```python
from build123d import *

# Parameters (mm, degrees)
F0_R           = 6.4699981168
F1_DEPTH       = 10
F1_DEPTH_BACK  = 50
F1_FACE_R      = 6.4699981168
F2_DEPTH       = 5
F2_TAPER       = 10
F1_FACE1_R     = 6.4699981168
F3_DEPTH       = 5
F3_TAPER       = 10
F4_R           = 2.6340165395
F5_DEPTH       = 5
F5_TAPER       = -20
F6_R           = 3.8875838451
F7_DEPTH       = 5
F7_TAPER       = 20
F8_W           = 10.0221466273
F8_H           = 2.0072241314
F8_H_2         = 1.9136306364
F8_W_2         = 10.0826621056
F9_DEPTH       = 25
F10_R          = 6.2562819227
F11_DEPTH      = 10
F11_DEPTH_BACK = 50
F11_FACE_R     = 6.2562819227
F12_DEPTH      = 5
F12_TAPER      = 10
F11_FACE1_R    = 6.2562819227
F13_DEPTH      = 5
F13_TAPER      = 10
F14_R          = 2.2911639189
F15_DEPTH      = 5
F15_TAPER      = -20
F16_R          = 3.8569980959
F17_DEPTH      = 5
F17_TAPER      = 20
F18_R          = 6.6968336437
F19_DEPTH      = 10
F19_DEPTH_BACK = 50
F19_FACE_R     = 6.6968336437
F20_DEPTH      = 5
F20_TAPER      = 10
F19_FACE1_R    = 6.6968336437
F21_DEPTH      = 5
F21_TAPER      = 10
F22_R          = 2.6922121505
F23_DEPTH      = 5
F23_TAPER      = -20
F24_R          = 3.9459371666
F25_DEPTH      = 5
F25_TAPER      = 20
F26_DEPTH      = 30
F26_FACE_R     = 5.5883632132
F27_DEPTH      = 5
F27_TAPER      = -10
F28_DEPTH      = 10
F28_FACE_R     = 6.4699981168
F29_DEPTH      = 5
F29_TAPER      = 10
F29_FACE_R     = 5.5883632132
F30_DEPTH      = 3
F30_TAPER      = 15
F30_FACE_R     = 4.7845156359
F31_DEPTH      = 2
F31_TAPER      = 40
F31_FACE_R     = 3.1063163736
F32_DEPTH      = 1
F32_TAPER      = 50
F33_DEPTH      = 10
F33_FACE_R     = 1.914562781
F34_DEPTH      = 3
F34_TAPER      = 30


with BuildPart() as f1:
    # F0 (on Top) → F1 (new body, two sides)
    with BuildSketch(Plane.XY) as f1_sk:
        Circle(F0_R)
    extrude(amount=F1_DEPTH)
    extrude(f1_sk.sketch, amount=-F1_DEPTH_BACK)

    # F1_face (on face) → F2 (join)
    with BuildSketch(Plane.XY.offset(10)):
        Circle(F1_FACE_R)
    extrude(amount=F2_DEPTH, taper=F2_TAPER)

    # F1_face1 (on face) → F3 (join)
    with BuildSketch(Plane(origin=(0, 0, -50), x_dir=(1, 0, 0), z_dir=(0, 0, -1))):
        Circle(F1_FACE1_R)
    extrude(amount=F3_DEPTH, taper=F3_TAPER)

    # F4 (on face) → F5 (join)
    with BuildSketch(Plane(origin=(0, 0, -55), x_dir=(1, 0, 0), z_dir=(0, 0, -1))):
        Circle(F4_R)
    extrude(amount=F5_DEPTH, taper=F5_TAPER)

    # F6 (on face) → F7 (cut)
    with BuildSketch(Plane(origin=(0, 0, -60), x_dir=(1, 0, 0), z_dir=(0, 0, -1))):
        Circle(F6_R)
    extrude(amount=-F7_DEPTH, taper=F7_TAPER, mode=Mode.SUBTRACT)

    # F8 (on Top) → F9 (join)
    with BuildSketch(Plane.XY):
        with Locations((-5.0110733137, -1.0036120657)):
            Rectangle(F8_W, F8_H)
        with Locations((-5.0110733137, 0.9568153182)):
            Rectangle(F8_W, F8_H_2)
        with Locations((5.0413310528, 0.9568153182)):
            Rectangle(F8_W_2, F8_H_2)
        with Locations((5.0413310528, -1.0036120657)):
            Rectangle(F8_W_2, F8_H)
    extrude(amount=-F9_DEPTH)

    # F10 (on face) → F11 (join, two sides)
    with BuildSketch(Plane.XY) as f11_sk:
        with BuildLine():
            ThreePointArc((9.3005501419, -2.0072241314), (16.2432425413, -6.1730446317), (21.4823797001, 0))
            ThreePointArc((21.4823797001, 0), (16.1945878695, 6.1808648616), (9.269665852, 1.9136306364))
            Line((9.269665852, 1.9136306364), (10.0826621056, 1.9136306364))
            Line((10.0826621056, 1.9136306364), (10.0826621056, -2.0072241314))
            Line((10.0826621056, -2.0072241314), (9.3005501419, -2.0072241314))
        make_face()
        with Locations((15.2260977775, 0)):
            Circle(F10_R)
    extrude(amount=F11_DEPTH)
    extrude(f11_sk.sketch, amount=-F11_DEPTH_BACK)

    # F11_face (on face) → F12 (join)
    with BuildSketch(Plane(origin=(15.2260977775, 0, 10), x_dir=(1, 0, 0), z_dir=(0, 0, 1))):
        Circle(F11_FACE_R)
    extrude(amount=F12_DEPTH, taper=F12_TAPER)

    # F11_face1 (on face) → F13 (join)
    with BuildSketch(Plane(origin=(15.2260977775, 0, -50), x_dir=(1, 0, 0), z_dir=(0, 0, -1))):
        Circle(F11_FACE1_R)
    extrude(amount=F13_DEPTH, taper=F13_TAPER)

    # F14 (on face) → F15 (join)
    with BuildSketch(Plane(origin=(0, 0, -55), x_dir=(1, 0, 0), z_dir=(0, 0, -1))):
        with Locations((15.2260977775, 0)):
            Circle(F14_R)
    extrude(amount=F15_DEPTH, taper=F15_TAPER)

    # F16 (on face) → F17 (cut)
    with BuildSketch(Plane(origin=(0, 0, -60), x_dir=(1, 0, 0), z_dir=(0, 0, -1))):
        with Locations((15.2260977775, 0)):
            Circle(F16_R)
    extrude(amount=-F17_DEPTH, taper=F17_TAPER, mode=Mode.SUBTRACT)

    # F18 (on face) → F19 (join, two sides)
    with BuildSketch(Plane.XY) as f19_sk:
        with BuildLine():
            ThreePointArc((-8.7388105431, -2.0072241314), (-8.5083423849, -1.0153501193), (-8.4309229892, 0))
            ThreePointArc((-8.4309229892, 0), (-8.5010989129, 0.9669479373), (-8.7101559411, 1.9136306364))
            Line((-8.7101559411, 1.9136306364), (-10.0221466273, 1.9136306364))
            Line((-10.0221466273, 1.9136306364), (-10.0221466273, -2.0072241314))
            Line((-10.0221466273, -2.0072241314), (-8.7388105431, -2.0072241314))
        make_face()
        with Locations((-15.1277566329, 0)):
            Circle(F18_R)
    extrude(amount=F19_DEPTH)
    extrude(f19_sk.sketch, amount=-F19_DEPTH_BACK)

    # F19_face (on face) → F20 (join)
    with BuildSketch(Plane(origin=(-15.1277566329, 0, 10), x_dir=(1, 0, 0), z_dir=(0, 0, 1))):
        Circle(F19_FACE_R)
    extrude(amount=F20_DEPTH, taper=F20_TAPER)

    # F19_face1 (on face) → F21 (join)
    with BuildSketch(Plane(origin=(-15.1277566329, 0, -50), x_dir=(1, 0, 0), z_dir=(0, 0, -1))):
        Circle(F19_FACE1_R)
    extrude(amount=F21_DEPTH, taper=F21_TAPER)

    # F22 (on face) → F23 (join)
    with BuildSketch(Plane(origin=(0, 0, -55), x_dir=(1, 0, 0), z_dir=(0, 0, -1))):
        with Locations((-15.1277566329, 0)):
            Circle(F22_R)
    extrude(amount=F23_DEPTH, taper=F23_TAPER)

    # F24 (on face) → F25 (cut)
    with BuildSketch(Plane(origin=(0, 0, -60), x_dir=(1, 0, 0), z_dir=(0, 0, -1))):
        with Locations((-15.1277566329, 0)):
            Circle(F24_R)
    extrude(amount=-F25_DEPTH, taper=F25_TAPER, mode=Mode.SUBTRACT)

    # F26 (add): a face of the model
    f26_faces = [f1.faces().sort_by_distance(p)[0] for p in [
        (0, 0, 15),
    ]]
    extrude(f26_faces, amount=F26_DEPTH)

    # F26_face (on face) → F27 (join)
    with BuildSketch(Plane.XY.offset(45)):
        Circle(F26_FACE_R)
    extrude(amount=F27_DEPTH, taper=F27_TAPER)

    # F28 (add): a face of the model
    f28_faces = [f1.faces().sort_by_distance(p)[0] for p in [
        (0, 0, 50),
    ]]
    extrude(f28_faces, amount=F28_DEPTH)

    # F28_face (on face) → F29 (join)
    with BuildSketch(Plane.XY.offset(60)):
        Circle(F28_FACE_R)
    extrude(amount=F29_DEPTH, taper=F29_TAPER)

    # F29_face (on face) → F30 (join)
    with BuildSketch(Plane.XY.offset(65)):
        Circle(F29_FACE_R)
    extrude(amount=F30_DEPTH, taper=F30_TAPER)

    # F30_face (on face) → F31 (join)
    with BuildSketch(Plane.XY.offset(68)):
        Circle(F30_FACE_R)
    extrude(amount=F31_DEPTH, taper=F31_TAPER)

    # F31_face (on face) → F32 (join)
    with BuildSketch(Plane.XY.offset(70)):
        Circle(F31_FACE_R)
    extrude(amount=F32_DEPTH, taper=F32_TAPER)

    # F33 (add): a face of the model
    f33_faces = [f1.faces().sort_by_distance(p)[0] for p in [
        (0, 0, 71),
    ]]
    extrude(f33_faces, amount=F33_DEPTH)

    # F33_face (on face) → F34 (join)
    with BuildSketch(Plane.XY.offset(81)):
        Circle(F33_FACE_R)
    extrude(amount=F34_DEPTH, taper=F34_TAPER)


solid = f1.part
```
Geometry check sheet. Reference: the model listing, model coordinates, mm. A direction names the side the tool comes from. Round coordinates to 2 decimals unless told otherwise and drop trailing zeros. Order: outer loops, then holes, each group sorted by start corner. A loop starts at its lowest first (then second) coordinate and runs counter-clockwise, first axis right, second up. Notation, with made-up numbers: (-14.5, -4) - (30.5, -4) arc R17 cw to (30.5, 15) - close; hole circle Ø7 at (22, -3). An arc over 180 degrees is marked (long way). Use a Markdown table: item, result. Add a question column.
1) Section check B-B (z = 25). Record the cut outline in (x, y).
2) Set-up check for faces 4 (the flat face through (15, 0, 15)), 5 (the cylindrical face through (-0.25, -1.9, 75.93)), 6 (the flat face through (18, 0, -55)): record each of +Z, -Z, +X, -X, +Y, -Y from which the full face is reachable in a straight line by a thin tool's end or side.
3) Mould release check, pull along Z, two halves, no side actions. Record for faces 1 (the flat face through (-7, -2.007, -12)), 2 (the conical face through (-0.555, 2.5, -56.354)), 3 (the flat face through (-14, 3, -55)): released by +Z, released by -Z, zero draft, split by the parting line, or undercut.
4) Section check A-A (z = -16). Record the cut outline in (x, y).
5) Gauge pin test, flat ends, axial feed: P1, Ø4, axis at y = -4.5, z = -1.5, coming from the +X side; P2, Ø1.6, axis at x = 8, y = -0.5, coming from the +Z side; P3, Ø1.5, axis at x = -12, y = 4.5, coming from the +Z side; P4, Ø8, axis at x = 9.5, y = 3, coming from the -Z side. Record the tip position at first contact, or that the pin passes through.
6) Thickness scan on line 1 along X through (y, z) = (-0.5, -44); line 2 along X through (y, z) = (-3, -47.5); line 3 along Z through (x, y) = (-12, 2.5). Record the ranges inside material, lowest first.
Established:
| question | item | result |
|---|---|---|
| 1 | outline | circle Ø11.18 at (0, 0) |
| 2 | face 4 | +Z, +X, +Y, -Y |
| 2 | face 5 | +Z |
| 2 | face 6 | none |
| 3 | face 1 | zero draft |
| 3 | face 2 | released by -Z |
| 3 | face 3 | undercut |
| 4 | outline | (-8.74, -2.01) - (-6.15, -2.01) arc R6.47 ccw to (6.15, -2.01) - (9.3, -2.01) arc R6.26 ccw (long way) to (9.27, 1.91) - (6.18, 1.91) arc R6.47 ccw to (-6.18, 1.91) - (-8.71, 1.91) arc R6.7 ccw (long way) to start |
| 5 | P1 | x = 20.96 |
| 5 | P2 | z = 0 |
| 5 | P3 | z = 15 |
| 5 | P4 | z = -60 |
| 6 | line 1 | -21.81 to -8.45, -6.45 to 6.45, 8.99 to 21.46 |
| 6 | line 2 | -21.12 to -9.14, -5.73 to 5.73, 9.74 to 20.72 |
| 6 | line 3 | -60 to -58.6, -55 to 15 |
